Could you check a few things on this model? Use its own coordinates, in mm. Coordinates: 2 decimals unless noted, no trailing zeros. Loops run counter-clockwise (first coordinate to the right, second up) from the corner with the lowest first, then second, coordinate; pieces in that order, holes last. Notation, with made-up numbers: (74, -12) -> (133, -12) arc R17 cw to (133, 18) -> close; hole circle Ø2 at (67, -12.75). An arc over 180 degrees is marked (long way). One line per question, with ' | ' between items.
Autodesk Inventor part; units mm, degrees
ref_plane "YZ Plane" through (0, 0, 0) normal (1, 0, 0) x (0, 1, 0)
ref_plane "XZ Plane" through (0, 0, 0) normal (0, 1, 0) x (-1, 0, 0)
ref_plane "XY Plane" through (0, 0, 0) normal (0, 0, 1) x (1, 0, 0)
sketch "Sketch1" plane through (0, 0, 0) normal (0, 0, 1) x (1, 0, 0)
  line L0 (-145, -145) -> (145, -145)
  line L1 (145, -145) -> (145, 145)
  line L2 (145, 145) -> (-145, 145)
  line L3 (-145, 145) -> (-145, -145)
  line L4 (-145, -145) -> (145, 145) construction
  line L5 (145, -145) -> (-145, 145) construction
  point P0 (0, 0)
  dimension "d0" = 290
  dimension "d1" = 290
extrude "Extrusion1" add sketch "Sketch1" along normal blind 5
sketch "Sketch2" plane through (0, 0, 5) normal (0, 0, 1) x (1, 0, 0)
  line L0 (-137.5, -137.5) -> (137.5, -137.5) construction
  line L1 (137.5, -137.5) -> (137.5, 137.5) construction
  line L2 (137.5, 137.5) -> (-137.5, 137.5) construction
  line L3 (-137.5, 137.5) -> (-137.5, -137.5) construction
  line L4 (-137.5, -137.5) -> (137.5, 137.5) construction
  line L5 (137.5, -137.5) -> (-137.5, 137.5) construction
  point P0 (0, 0)
  dimension "d4" = 275
  dimension "d5" = 275
hole "Hole1" at (-137.5, 137.5, 5) at (137.5, 137.5, 5) at (137.5, -137.5, 5) at (-137.5, -137.5, 5) direction (0, 0, -1) diameter 5.5 depth 8 tip angle 118
fillet "Fillet1" radius 6 4 edges at (145, -145, 2.5) (-145, -145, 2.5) (145, 145, 2.5) (-145, 145, 2.5)
sketch "Sketch3" plane through (0, 0, 5) normal (0, 0, 1) x (1, 0, 0)
  line L0 (-110, -20.75) -> (-20, -20.75) construction
  line L1 (-20, -20.75) -> (-20, 28.75) construction
  line L2 (-20, 28.75) -> (-110, 28.75) construction
  line L3 (-110, 28.75) -> (-110, -20.75) construction
  line L4 (-139, -145) -> (139, -145)
  arc A0 (-139, 145) -> (-145, 139) centre (-139, 139) ccw
  line L5 (-145, 139) -> (-145, -139)
  arc A1 (-145, -139) -> (-139, -145) centre (-139, -139) ccw
  line L6 (-139, -145) -> (139, -145)
  arc A2 (139, -145) -> (145, -139) centre (139, -139) ccw
  line L7 (145, -139) -> (145, 139)
  arc A3 (145, 139) -> (139, 145) centre (139, 139) ccw
  line L8 (139, 145) -> (-139, 145)
  circle A4 centre (137.5, -137.5) radius 2.75
  circle A5 centre (-137.5, 137.5) radius 2.75
  circle A6 centre (137.5, 137.5) radius 2.75
  circle A7 centre (-137.5, -137.5) radius 2.75
  line L9 (-110, -90.25) -> (-20, -90.25) construction
  line L10 (-20, -90.25) -> (-20, -40.75) construction
  line L11 (-20, -40.75) -> (-110, -40.75) construction
  line L12 (-110, -40.75) -> (-110, -90.25) construction
  line L13 (20, -55.5) -> (110, -55.5) construction
  line L14 (110, -55.5) -> (110, -6) construction
  line L15 (110, -6) -> (20, -6) construction
  line L16 (20, -6) -> (20, -55.5) construction
  line L17 (-110, 48.75) -> (-20, 48.75) construction
  line L18 (-20, 48.75) -> (-20, 98.25) construction
  line L19 (-20, 98.25) -> (-110, 98.25) construction
  line L20 (-110, 98.25) -> (-110, 48.75) construction
  line L21 (20, -125) -> (110, -125) construction
  line L22 (110, -125) -> (110, -75.5) construction
  line L23 (110, -75.5) -> (20, -75.5) construction
  line L24 (20, -75.5) -> (20, -125) construction
  line L25 (20, 14) -> (110, 14) construction
  line L26 (110, 14) -> (110, 63.5) construction
  line L27 (110, 63.5) -> (20, 63.5) construction
  line L28 (20, 63.5) -> (20, 14) construction
  point P0 (0, 0)
  point P1 (-20, 73.5)
  point P2 (20, 38.75)
  point P3 (20, -30.75)
  point P4 (-20, -65.5)
  point P5 (20, -100.25)
  point P6 (-20, 4)
  dimension "d14" = 49.5
  dimension "d16" = 49.5
  dimension "d17" = 90
  dimension "d20" = 49.5
  dimension "d25" = 90
  dimension "d26" = 290
  dimension "d29" = 20
  dimension "d71" = 49.5
  dimension "d72" = 49.5
  dimension "d73" = 49.5
  dimension "d75" = 20
  dimension "d76" = 20
  dimension "d77" = 20
  dimension "d78" = 54.75
  dimension "d79" = 20
  dimension "d81" = 40
  dimension "d82" = 35
hole "Hole2" at (-20, 73.5, 5) at (20, 38.75, 5) at (20, -30.75, 5) at (-20, -65.5, 5) at (20, -100.25, 5) at (110, 63.5, 5) at (110, 14, 5) at (110, -6, 5) at (110, -55.5, 5) at (110, -75.5, 5) at (110, -125, 5) at (-110, -40.75, 5) at (-110, -90.25, 5) at (-110, -20.75, 5) at (-110, 28.75, 5) at (-110, 48.75, 5) at (-110, 98.25, 5) at (-20, 4, 5) direction (0, 0, -1) diameter 3.4 end through all
sketch "Sketch4" plane through (0, 0, 5) normal (0, 0, 1) x (1, 0, 0)
  line L0 (-120, -140) -> (120, -140)
  line L1 (120, -140) -> (120, -135)
  line L2 (120, -135) -> (-120, -135)
  line L3 (-120, -135) -> (-120, -140)
  line L4 (140, -120) -> (135, -120)
  line L5 (135, -120) -> (135, 120)
  line L6 (135, 120) -> (140, 120)
  line L7 (140, 120) -> (140, -120)
  line L8 (120, 140) -> (-120, 140)
  line L9 (-120, 140) -> (-120, 135)
  line L10 (-120, 135) -> (120, 135)
  line L11 (120, 135) -> (120, 140)
  line L12 (-135, 120) -> (-140, 120)
  line L13 (-140, 120) -> (-140, -120)
  line L14 (-140, -120) -> (-135, -120)
  line L15 (-135, -120) -> (-135, 120)
  line L16 (-139, -145) -> (139, -145)
  line L17 (-145, 139) -> (-145, -139)
  line L18 (139, 145) -> (-139, 145)
  line L19 (145, -139) -> (145, 139)
  point P0 (0, 0)
  point P1 (0, -140)
  point P2 (-140, 0)
  point P3 (140, 0)
  point P4 (0, 140)
  dimension "d39" = 5
  dimension "d40" = 5
  dimension "d41" = 5
  dimension "d42" = 5
  dimension "d43" = 240
  dimension "d44" = 240
  dimension "d45" = 240
  dimension "d46" = 5
  dimension "d47" = 5
  dimension "d48" = 5
  dimension "d49" = 5
extrude "Extrusion2" cut sketch "Sketch4" against normal through all
sketch "Sketch5" plane through (0, 0, 5) normal (0, 0, 1) x (1, 0, 0)
  point P0 (0, 0)
  point P1 (120, 0)
  dimension "d60" = 120
hole "Hole3" at (120, 0, 5) direction (0, 0, -1) diameter 8 depth 8 tip angle 118
sketch "Sketch7" plane through (0, 0, 5) normal (0, 0, 1) x (1, 0, 0)
  point P0 (0, 0)
  point P1 (85, 105)
  dimension "d85" = 85
  dimension "d102" = 105
hole "Hole5" at (85, 105, 5) direction (0, 0, -1) diameter 3.4 depth 8 tip angle 118
sketch "Sketch8" plane through (0, 0, 5) normal (0, 0, 1) x (1, 0, 0)
  circle A0 centre (85, 105) radius 1.7
  point P0 (0, 0)
  point P1 (66.5, 123)
  dimension "d108" = 18
  dimension "d118" = 18.5
hole "Hole6" at (66.5, 123, 5) direction (0, 0, -1) diameter 8 depth 8 tip angle 118
sketch "Sketch6" plane through (0, 0, 5) normal (0, 0, 1) x (1, 0, 0)
  line L0 (139, 145) -> (-139, 145)
  point P0 (0, 0)
  point P1 (0, 120)
  dimension "d107" = 120
hole "Hole4" at (0, 120, 5) direction (0, 0, -1) diameter 12 depth 8 tip angle 118
sketch "Sketch9" plane through (0, 0, 5) normal (0, 0, 1) x (1, 0, 0)
  circle A0 centre (85, 105) radius 1.7
  point P0 (0, 0)
  point P1 (103.5, 87)
  dimension "d109" = 18
  dimension "d110" = 18.5
hole "Hole7" at (103.5, 87, 5) direction (0, 0, -1) diameter 12 end through all
properties part number "mid" material "Polycarbonate, Clear"
1) If we section it at A-A on x = 74: Please give me the cut outline in (y, z).
Data:
outline: (-145, 0) -> (-140, 0) -> (-140, 5) -> (-145, 5) -> close; (-135, 0) -> (135, 0) -> (135, 5) -> (-135, 5) -> close; (140, 0) -> (145, 0) -> (145, 5) -> (140, 5) -> close
2) If we section it at C-C on z = 2.1: Give the number of separate pieces and of enclosed holes in the cut face, and give its area (3 significant figures).
Data:
separate pieces: 1 | enclosed holes: 31 | area: 78,700 mm²
3) I need wall thicknesses on line 1 along Y through (x, z) = (-95, 3.8); line 2 along X through (y, z) = (-6, 3.5). Which ranges of each line are inside material? Lowest first, please. Write a range as from..to.
Data:
line 1: -145..-140, -135..135, 140..145 | line 2: -145..-140, -135..108.3, 111.7..135, 140..145
4) I'm going to push a flat-ended pin straight in: pin 1 Ø2.5 at (x, y) = (-110, -90.25) entering from +Z. Where does the tip first touch, or does it pass through?
Data:
pin 1: through
5) We'd pull the mould along Y, two halves only. Please class faces 1 (the face through (-2, 2, 0)), 2 (the face through (97.55, 87.78, 2.46)): pulls with the +Y half, pulls with the -Y half, needs draft (parallel to the pull), parting line crosses it, or undercut.
Data:
face 1: needs draft | face 2: undercut
